Job drawing, mm, ordinate dimensions from the low corner. One solid piece. A direction names the side the tool comes from. Give positions to 0.01 mm unless a question says otherwise; leave off trailing zeros. Write each loop counter-clockwise with the first axis right and the second up, starting at its lowest first coordinate (ties: lowest second). Pieces come first, ordered by that corner, then holes. Notation, with made-up numbers: (34, 40) -> (65, 40) arc R15 cw to (65, 69) -> close; hole circle Ø7 at (-37, -28.75). An arc over 180 degrees is marked (long way). Put each result on its own line as item: value. Start each with the question number.
Item 1: Drill centre lines: line 1 along Z through (x, y) = (249, 70); line 2 along Y through (x, z) = (99, 70). Where is each one in solid material? Low to high.
Item 2: Tool access for the marked faces 1 and 2: list every direction of +Z, -Z, +X, -X, +Y, -Y with a clear straight run to the whole face (end or side of a thin tool).
Item 3: Slice it at C-C, the plane x = 233. List the corners of the cut face in (y, z), plus the area to 3 significant figures.
Item 4: Slice it at D-D, the plane x = 30. List the corners of the cut face in (y, z).
Item 5: Flat gauge pins, fed straight in: pin 1 Ø10 at (x, z) = (57, 47) entering from -Y; pin 2 Ø10 at (x, y) = (323.5, 73.5) entering from -Z; pin 3 Ø3 at (x, y) = (389, 20) entering from +Z; pin 4 Ø8 at (x, z) = (278, 47) entering from +Y. Where does each tip first touch, or does it go through?
Item 6: Slice it at A-A, the plane y = 70. List the corners of the cut face in (x, z).
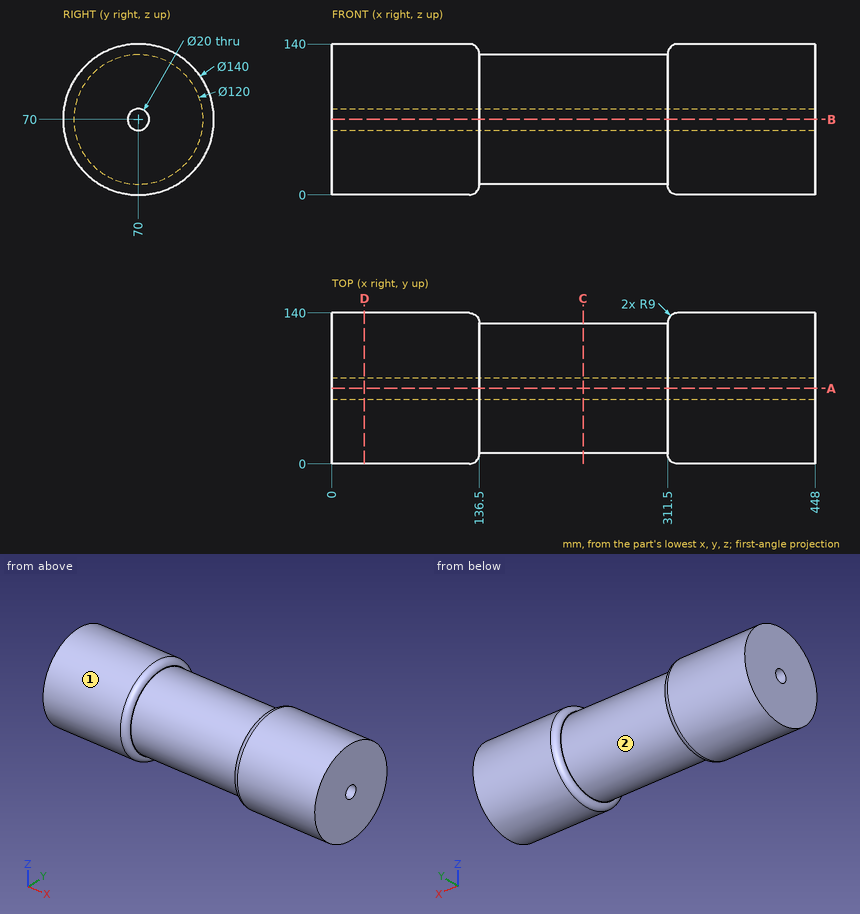
Values follow:
1. line 1: 10 to 60, 80 to 130
1. line 2: 0 to 60, 80 to 140
2. face 1: +X, -X
2. face 2: none
3. outline: circle Ø120 at (70, 70); hole circle Ø20 at (70, 70)
3. area: 11,000 mm2
4. outline: circle Ø140 at (70, 70); hole circle Ø20 at (70, 70)
5. pin 1: y = 2.35
5. pin 2: z = 0
5. pin 3: z = 120.48
5. pin 4: y = 126.91
6. outline: (0, 0) -> (127.5, 0) arc R9 ccw to (136.5, 9) -> (136.5, 10) -> (311.5, 10) -> (311.5, 9) arc R9 ccw to (320.5, 0) -> (448, 0) -> (448, 60) -> (0, 60) -> close; (0, 80) -> (448, 80) -> (448, 140) -> (320.5, 140) arc R9 ccw to (311.5, 131) -> (311.5, 130) -> (136.5, 130) -> (136.5, 131) arc R9 ccw to (127.5, 140) -> (0, 140) -> close
